```python
from build123d import *

# Parameters (mm, degrees)
BOX_W          = 25
BOX_H          = 10
BOX_DEPTH      = 30
CYLINDER_R     = 10.125
CYLINDER_DEPTH = 25


with BuildPart() as obj1:
    # Box → Box (new body)
    with BuildSketch(Plane(origin=(-12.5, 7.7, -3), x_dir=(1, 0, 0), z_dir=(0, 0, 1))):
        with Locations((12.5, 5)):
            Rectangle(BOX_W, BOX_H)
    extrude(amount=BOX_DEPTH)


with BuildPart() as obj2:
    # Part__Mirroring: instance of obj1
    add(obj1.part.mirror(Plane(origin=(0, 0, 0), x_dir=(1, 0, 0), z_dir=(0, 1, 0))))

    # Fusion: union obj1
    add(obj1.part)


with BuildPart() as master_cuerpo_motor_con_offset_0_2_mm:
    # Cylinder → Cylinder (new body)
    with BuildSketch(Plane.XY):
        Circle(CYLINDER_R)
    extrude(amount=CYLINDER_DEPTH)

    # Cut: cut obj2
    add(obj2.part, mode=Mode.SUBTRACT)


solid = master_cuerpo_motor_con_offset_0_2_mm.part
```
Input: part model. Units: mm. Frame: model coordinates. Coordinates: 2 decimals unless noted, no trailing zeros. Write each loop counter-clockwise with the first axis right and the second up, starting at its lowest first coordinate (ties: lowest second). Pieces come first, ordered by that corner, then holes.
1) Pin query (flat end, axial travel): pin 1 Ø1 at (y, z) = (1, 2.5) entering from -X; pin 2 Ø5 at (y, z) = (-4.5, 20) entering from -X; pin 3 Ø4 at (y, z) = (-5, 20.5) entering from -X. Return the tip coordinate at first contact, or that it passes through.
2) Section A-A on z = 5.75. Output: boundary loops of the cut face in (x, y) (3 decimals).
3) Material intervals for line 1 along X through (y, z) = (-0.25, 7.75); line 2 along X through (y, z) = (4, 1.75); line 3 along Y through (x, z) = (-7.5, 9), sorted ascending.
4) Section B-B on y = 2.25. Output: boundary loops of the cut face in (x, z).
Check result:
1. pin 1: stops at x = -10.11
1. pin 2: stops at x = -9.93
1. pin 3: stops at x = -9.67
2. outline: (-6.575, -7.7) - (6.575, -7.7) arc R10.125 ccw to (6.575, 7.7) - (-6.575, 7.7) arc R10.125 ccw to start
3. line 1: x = -10.12 to 10.12
3. line 2: x = -9.3 to 9.3
3. line 3: y = -6.8 to 6.8
4. outline: (-9.87, 0) - (9.87, 0) - (9.87, 25) - (-9.87, 25) - close
